Here's how the part is built. I have some questions about the finished solid (model axes, mm). A direction names the side the tool comes from. Coordinates: 2 decimals unless noted, no trailing zeros. Write each loop counter-clockwise with the first axis right and the second up, starting at its lowest first coordinate (ties: lowest second). Pieces come first, ordered by that corner, then holes. Notation, with made-up numbers: M 39,38 L 54,38 A35 ccw 54,73 Z; hole C 61,12 d11. An arc over 180 degrees is marked long. Use one line per item in the form item = value. Start each with the question number.
1. Thinking about a two-plate mould opening in X: for faces 1 (the face through (-43.3, 19.4, 0)), 2 (the face through (-35.264, 11.718, 11.329)), which applies, released by +X, released by -X, zero draft, split by the parting line, or undercut?
2. On a 3-axis mill with a long thin cutter (end or side, diameter ignored), from which of +Z, -Z, +X, -X, +Y, -Y can I reach the whole of each face in a straight line? I mean faces 3 (the face through (-43.3, 19.4, 15.291)), 4 (the face through (-32.634, 14, 11)). Say none if no direction works.
3. Please list where these lines run through material, in increasing order: line 1 along X through (y, z) = (14.5, 12); line 2 along X through (y, z) = (12, 10.75); line 3 along Y through (x, z) = (-40, 2.5). Write a range as [from, to].
4. I want a section at B-B, the plane x = -46.75. List the corners of the cut face in (y, z) for me.
5. I want a section at D-D, the plane z = 10. List the corners of the cut face in (x, y) for me, plus the area to 3 significant figures.
6. I want a section at A-A, the plane y = 13.25. List the corners of the cut face in (x, z) for me, plus the area to 3 significant figures.
7. I want a section at C-C, the plane y = 9.75. List the corners of the cut face in (x, z) for me, plus the area to 3 significant figures.
8. I'm going to push flat-ended pins straight in: pin 1 Ø1 at (x, z) = (-40.5, 8) entering from -Y; pin 2 Ø5 at (x, z) = (-40.5, 12) entering from +Y; pin 3 Ø1 at (x, z) = (-40, 9) entering from +Y; pin 4 Ø6.5 at (x, y) = (-43.27, 13.76) entering from +Z. Where does each tip first touch, or does it pass through?
from build123d import *

# Parameters (mm, degrees)
F0_R          = 6.826248
F0_R_2        = 5.483861
F1_DEPTH      = 15.2908
F3_R          = 2.032
F4_DEPTH      = 2.8956
F4_DEPTH_BACK = 1.6256


with BuildPart() as f1:
    # F0 (on Top) → F1 (new body)
    with BuildSketch(Plane.XY):
        with Locations((-43.26782, 13.760585)):
            Circle(F0_R)
        with Locations((-43.26782, 13.760585)):
            Circle(F0_R_2, mode=Mode.SUBTRACT)
    extrude(amount=F1_DEPTH)

    # F3 (on offset) → F4 (join, two sides)
    with BuildSketch(Plane.YZ.offset(-35.52952)) as f4_sk:
        with Locations((13.747922, 11.24013)):
            Circle(F3_R)
    extrude(amount=F4_DEPTH)
    extrude(f4_sk.sketch, amount=-F4_DEPTH_BACK)

    # F5 (on face) → F6 (revolve)
    with BuildSketch(Plane.YZ.offset(-32.63392)):
        with BuildLine():
            Line((11.398422, 11.24013), (11.715922, 11.24013))
            ThreePointArc((11.715922, 11.24013), (13.747922, 13.27213), (15.779922, 11.24013))
            Line((15.779922, 11.24013), (16.097422, 11.24013))
            ThreePointArc((16.097422, 11.24013), (13.747922, 13.58963), (11.398422, 11.24013))
        make_face()
    revolve(axis=Axis((-32.63392, 12.573172, 11.24013), (0, -1, 0)))


solid = f1.part
Answer list:
q1.face_1 = zero draft
q1.face_2 = undercut
q2.face_3 = +Z, +X, -X, +Y, -Y
q2.face_4 = none
q3.line_1 = [-50.05, -48.7], [-37.83, -32.63], [-30.91, -30.54]
q3.line_2 = [-49.86, -48.46], [-38.07, -32.63], [-31.72, -31.14]
q3.line_3 = [7.77, 9.36], [18.16, 19.75]
q4.outline = M 7.89,0 L 9.52,0 L 9.52,15.29 L 7.89,15.29 Z; M 18,0 L 19.63,0 L 19.63,15.29 L 18,15.29 Z
q5.outline = M -36.64,12.14 L -33.81,12.14 A2 ccw long -33.81,15.36 L -36.63,15.36 A6.83 ccw long Z; hole C -43.27,13.76 d10.97; hole M -32.63,12.14 A1.61 ccw -32.63,15.36 Z
q5.area = 67.2 mm²
q6.outline = M -50.07,0 L -48.73,0 L -48.73,15.29 L -50.07,15.29 Z; M -37.81,0 L -36.46,0 L -36.46,9.27 L -33.81,9.27 A2.3 ccw long -33.81,13.21 L -36.46,13.21 L -36.46,15.29 L -37.81,15.29 Z; hole M -32.63,9.27 A1.97 ccw -32.63,13.21 Z
q6.area = 59.0 mm²
q7.outline = M -48.79,0 L -47.01,0 L -47.01,15.29 L -48.79,15.29 Z; M -39.53,0 L -37.74,0 L -37.74,15.29 L -39.53,15.29 Z
q7.area = 54.6 mm²
q8.pin_1 = 7.32
q8.pin_2 = 20.58
q8.pin_3 = 20
q8.pin_4 = through
